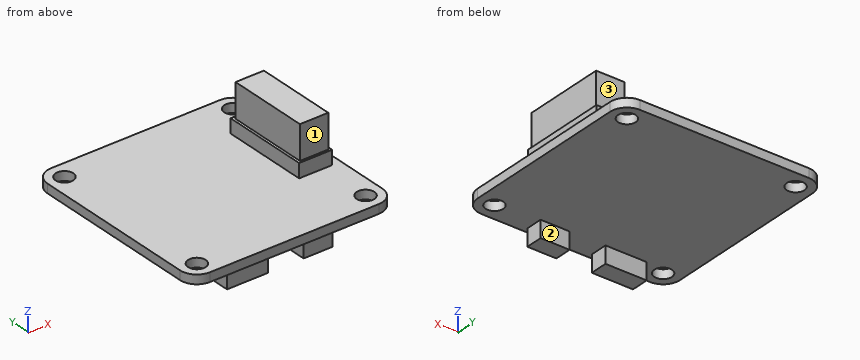
from build123d import *

# Parameters (mm, degrees)
F0_W     = 36
F0_H     = 36
F1_DEPTH = 1.6
F2_R     = 3
F3_D     = 3.15
F4_W     = 5.162462825
F4_H     = 2.9942281544
F4_W_2   = 7.3306979612
F4_H_2   = 3.097477369
F5_DEPTH = 3
F6_W     = 5.8629876003
F6_H     = 15.5157274567
F7_DEPTH = 2.5
F8_W     = 5.0398427993
F8_H     = 14.5735112019
F9_DEPTH = 6


with BuildPart() as f1:
    # F0 (on Top) → F1 (new body)
    with BuildSketch(Plane.XY):
        Rectangle(F0_W, F0_H)
    extrude(amount=-F1_DEPTH)

    # F2
    f2_edges = [f1.edges().sort_by_distance(p)[0] for p in [
        (18, -18, -0.8),
        (-18, -18, -0.8),
        (18, 18, -0.8),
        (-18, 18, -0.8),
    ]]
    fillet(f2_edges, radius=F2_R)

    # F3 (through all)
    with Locations(Plane.XY):
        with Locations((-15, 15), (15, 15), (15, -15), (-15, -15)):
            Hole(F3_D / 2)

    # F4 (on face) → F5 (join)
    with BuildSketch(Plane(origin=(0, 0, -1.6), x_dir=(1, 0, 0), z_dir=(0, 0, -1))):
        with Locations((4.9126524245, 15.6052540988)):
            Rectangle(F4_W, F4_H)
        with Locations((-7.6321330853, 15.5536294915)):
            Rectangle(F4_W_2, F4_H_2)
    extrude(amount=F5_DEPTH)

    # F6 (on face) → F7 (join)
    with BuildSketch(Plane.XY):
        with Locations((13.4858717211, 2.1426391322)):
            Rectangle(F6_W, F6_H)
    extrude(amount=F7_DEPTH)

    # F8 (on face) → F9 (join)
    with BuildSketch(Plane.XY.offset(2.5)):
        with Locations((13.5199902579, 2.0592806395)):
            Rectangle(F8_W, F8_H)
    extrude(amount=F9_DEPTH)


solid = f1.part
For this review, take the finished solid that the model builds, in its own axes (mm). Face numbers are marked on the shaded views. A direction names the side the tool comes from. Give positions to 0.01 mm unless a question says otherwise; leave off trailing zeros. Loops run counter-clockwise (first coordinate to the right, second up) from the corner with the lowest first, then second, coordinate; pieces in that order, holes last. Notation, with made-up numbers: (81, 18.5) -> (113, 18.5) arc R20 ccw to (113, 29.5) -> close; hole circle Ø6 at (37, 24.5). An arc over 180 degrees is marked (long way). One line per question, with ' | ' between items.
1) For the marked faces 1, 2 and 3, list the 3-axis set-ups (+Z, -Z, +X, -X, +Y, -Y) from which the entire face can be reached by the end or side of a thin tool; tool diameter is ignored.
Resolved:
face 1: +Z, +X, -X, -Y | face 2: -Z, +X, +Y | face 3: +Z, +X, -X, +Y
2) We need section D-D (z = 6.25). Write out the cut boundary in (x, y).
Resolved:
outline: (11, -5.23) -> (16.04, -5.23) -> (16.04, 9.35) -> (11, 9.35) -> close
3) Insertion check: pin 1 Ø2 at (y, z) = (-1, 4) entering from +X; pin 2 Ø5 at (x, y) = (-15, 15) entering from +Z; pin 3 Ø0.9 at (x, z) = (-8.5, -2.5) entering from +Y; pin 4 Ø2.5 at (x, y) = (-15, -15) entering from +Z. Each pin has a flat end and moves straight along its axis. Give the tip position at first contact, or say it passes through.
Resolved:
pin 1: stops at x = 16.04 | pin 2: stops at z = 0 | pin 3: stops at y = -14 | pin 4: passes through
4) We need section B-B (y = 6). Write out the cut boundary in (x, z), plus the area to 3 significant figures.
Resolved:
outline: (-18, -1.6) -> (18, -1.6) -> (18, 0) -> (16.42, 0) -> (16.42, 2.5) -> (16.04, 2.5) -> (16.04, 8.5) -> (11, 8.5) -> (11, 2.5) -> (10.55, 2.5) -> (10.55, 0) -> (-18, 0) -> close | area: 102 mm2
5) We need section A-A (z = -3.5). Write out the cut boundary in (x, y), plus the area to 3 significant figures.
Resolved:
outline: (-11.3, -17.1) -> (-3.97, -17.1) -> (-3.97, -14) -> (-11.3, -14) -> close; (2.33, -17.1) -> (7.49, -17.1) -> (7.49, -14.11) -> (2.33, -14.11) -> close | area: 38.2 mm2
6) We need section C-C (x = 13). Write out the cut boundary in (y, z).
Resolved:
outline: (-18, -1.6) -> (18, -1.6) -> (18, 0) -> (9.9, 0) -> (9.9, 2.5) -> (9.35, 2.5) -> (9.35, 8.5) -> (-5.23, 8.5) -> (-5.23, 2.5) -> (-5.62, 2.5) -> (-5.62, 0) -> (-18, 0) -> close
7) To check wall thickness, follow probe 1 along Y at (x, z) = (15, -0.6) (3 decimals); probe 2 along Y at (x, z) = (3, -3); probe 3 along Z at (x, y) = (10.5, -1.5). State the ranges of each line that lie inside material, in increasing order.
Resolved:
probe 1: y = -18 to -16.575, -13.425 to 13.425, 16.575 to 18 | probe 2: y = -17.1 to -14.11 | probe 3: z = -1.6 to 0
